The model under review builds one solid part; all positions refer to its coordinate system, in mm. A direction names the side the tool comes from. Coordinates: 2 decimals unless noted, no trailing zeros. Loops run counter-clockwise (first coordinate to the right, second up) from the corner with the lowest first, then second, coordinate; pieces in that order, holes last. Notation, with made-up numbers: (-5.75, 42.5) - (7.25, 42.5) arc R18 ccw to (7.25, 67.5) - close; hole circle Ø4 at (58.25, 73.5). An arc over 180 degrees is marked (long way). Use a Markdown table: item, result. Add a question column.
1) Add section B-B, the plane z = -12. Give the boundary of the cut face in (x, y), and give its area (3 significant figures).
2) Clearance check with flat-ended pins moving along their axes: pin 1 (6.5 mm diameter, centred on x = 25, z = -12, fed in from +Y); pin 2 (8 mm diameter, centred on x = 25, y = 12, fed in from -Z). State where each tip first meets the part, or that it passes through.
3) The part is to be moulded in two halves that separate along Y. For faces 3 (the cylindrical face through (9.46, 9.56, -1.97)), 4 (the cylindrical face through (24.46, 9.56, -1.97)), 5 (the flat face through (25, 20, -2)), 6 (the flat face through (50, 3, -5)), say which applies: pulls with the +Y half, pulls with the -Y half, needs draft (parallel to the pull), parting line crosses it, or undercut.
4) Add section D-D, the plane x = 45. Give the boundary of the cut face in (y, z).
5) Add section A-A, the plane x = 40. Give the boundary of the cut face in (y, z), and give its area (3 significant figures).
6) Add section C-C, the plane z = -3. Give the boundary of the cut face in (x, y), and give its area (3 significant figures).
7) For faces 1 (the flat face through (25, 8, 0)), 2 (the flat face through (25, 8, -4)), list the 3-axis set-ups (+Z, -Z, +X, -X, +Y, -Y) from which the entire face can be reached by the end or side of a thin tool; tool diameter is ignored.
8) To check wall thickness, follow L1, parallel to X at y = 3.2, z = -12; L2, parallel to Y at x = 25, z = -2.85; L3, parallel to X at y = 3, z = -14.25. State the ranges of each line that lie inside material, in increasing order. Write a range as [from, to].
```python
from build123d import *

# Parameters (mm, degrees)
SKETCH_1_W          = 50
SKETCH_1_H          = 20
SKETCH_1_R          = 2.5
EXTRUDE_1_DEPTH     = 4
SKETCH_2_W          = 50
SKETCH_2_H          = 4
EXTRUDE_2_DEPTH     = 16
SKETCH_3_R          = 2.5
CUT_EXTRUDE_1_DEPTH = 4


with BuildPart() as part:
    # Эскиз1 → Бобышка-Вытянуть1 (new body)
    with BuildSketch(Plane(origin=(0, 0, 0), x_dir=(1, 0, 0), z_dir=(0, 1, 0))):
        with Locations((25, 10)):
            Rectangle(SKETCH_1_W, SKETCH_1_H)
        with Locations(Location((10, 12, 0), (0, 0, 270))):
            Circle(SKETCH_1_R, mode=Mode.SUBTRACT)
        with Locations(Location((40, 12, 0), (0, 0, 270))):
            Circle(SKETCH_1_R, mode=Mode.SUBTRACT)
        with Locations(Location((25, 12, 0), (0, 0, 270))):
            Circle(SKETCH_1_R, mode=Mode.SUBTRACT)
    extrude(amount=EXTRUDE_1_DEPTH)

    # Эскиз2 → Бобышка-Вытянуть2 (add)
    with BuildSketch(Plane(origin=(0, 4, 0), x_dir=(1, 0, 0), z_dir=(0, 1, 0))):
        with Locations((25, 2)):
            Rectangle(SKETCH_2_W, SKETCH_2_H)
    extrude(amount=EXTRUDE_2_DEPTH)

    # Эскиз3 → Вырез-Вытянуть1 (cut)
    with BuildSketch(Plane.XY):
        with Locations((10, 12)):
            Circle(SKETCH_3_R)
        with Locations((40, 12)):
            Circle(SKETCH_3_R)
        with Locations((25, 12)):
            Circle(SKETCH_3_R)
    extrude(amount=-CUT_EXTRUDE_1_DEPTH, mode=Mode.SUBTRACT)


solid = part.part
```
From the geometry:
| question | item | result |
|---|---|---|
| 1 | outline | (0, 0) - (7.5, 0) - (7.5, 4) - (0, 4) - close; (12.5, 0) - (22.5, 0) - (22.5, 4) - (12.5, 4) - close; (27.5, 0) - (37.5, 0) - (37.5, 4) - (27.5, 4) - close; (42.5, 0) - (50, 0) - (50, 4) - (42.5, 4) - close |
| 1 | area | 140 mm^2 |
| 2 | pin 1 | stops at y = 4 |
| 2 | pin 2 | stops at z = -4 |
| 3 | face 3 | undercut |
| 3 | face 4 | undercut |
| 3 | face 5 | pulls with the +Y half |
| 3 | face 6 | needs draft |
| 4 | outline | (0, -20) - (4, -20) - (4, -4) - (20, -4) - (20, 0) - (0, 0) - close |
| 5 | outline | (0, -20) - (4, -20) - (4, -14.5) - (0, -14.5) - close; (0, -9.5) - (4, -9.5) - (4, -4) - (9.5, -4) - (9.5, 0) - (0, 0) - close; (14.5, -4) - (20, -4) - (20, 0) - (14.5, 0) - close |
| 5 | area | 104 mm^2 |
| 6 | outline | (0, 0) - (50, 0) - (50, 20) - (0, 20) - close; hole circle Ø5 at (10, 12); hole circle Ø5 at (25, 12); hole circle Ø5 at (40, 12) |
| 6 | area | 941 mm^2 |
| 7 | face 1 | +Z, +X, -X, +Y, -Y |
| 7 | face 2 | -Z, +X, -X, +Y |
| 8 | L1 | x = [0, 7.5], [12.5, 22.5], [27.5, 37.5], [42.5, 50] |
| 8 | L2 | y = [0, 9.5], [14.5, 20] |
| 8 | L3 | x = [0, 8.91], [11.09, 23.91], [26.09, 38.91], [41.09, 50] |
